Part model, mm, in its own coordinate system. A direction names the side the tool comes from. Round coordinates to 2 decimals unless told otherwise and drop trailing zeros.
```python
from build123d import *

# Parameters (mm, degrees)
F0_R     = 11.025
F1_DEPTH = 7
F2_R     = 1.5


with BuildPart() as f1:
    # F0 (on Top) → F1 (new body)
    with BuildSketch(Plane.XY):
        with BuildLine():
            Line((8.85511, 24.849853), (8.85511, 35.074853))
            Line((8.85511, 35.074853), (0, 40.187353))
            Line((0, 40.187353), (-8.85511, 35.074853))
            Line((-8.85511, 35.074853), (-8.85511, 24.849853))
            ThreePointArc((-8.85511, 24.849853), (-12.204102, 7.046041), (-25.948159, -4.756177))
            Line((-25.948159, -4.756177), (-34.803269, -9.868677))
            Line((-34.803269, -9.868677), (-34.803269, -20.093677))
            Line((-34.803269, -20.093677), (-25.948159, -25.206177))
            Line((-25.948159, -25.206177), (-17.093049, -20.093677))
            ThreePointArc((-17.093049, -20.093677), (0, -14.092083), (17.093049, -20.093677))
            Line((17.093049, -20.093677), (25.948159, -25.206177))
            Line((25.948159, -25.206177), (34.803269, -20.093677))
            Line((34.803269, -20.093677), (34.803269, -9.868677))
            Line((34.803269, -9.868677), (25.948159, -4.756177))
            ThreePointArc((25.948159, -4.756177), (12.204102, 7.046041), (8.85511, 24.849853))
        make_face()
        Polygon((-32.205193, -11.368677), (-25.948159, -7.756177), (-19.691126, -11.368677), (-19.691126, -18.593677), (-25.948159, -22.206177), (-32.205193, -18.593677), align=None, mode=Mode.SUBTRACT)
        Polygon((25.948159, -22.206177), (19.691126, -18.593677), (19.691126, -11.368677), (25.948159, -7.756177), (32.205193, -11.368677), (32.205193, -18.593677), align=None, mode=Mode.SUBTRACT)
        Circle(F0_R, mode=Mode.SUBTRACT)
        Polygon((0, 37.187353), (6.257034, 33.574853), (6.257034, 26.349853), (0, 22.737353), (-6.257034, 26.349853), (-6.257034, 33.574853), align=None, mode=Mode.SUBTRACT)
    extrude(amount=F1_DEPTH)

    # F2
    f2_edges = [f1.edges().sort_by_distance(p)[0] for p in [
        (0, -14.092083, 7),
        (-21.520604, -22.649927, 7),
        (-30.375714, -22.649927, 7),
        (-34.803269, -14.981177, 7),
        (-30.375714, -7.312427, 7),
        (-12.204102, 7.046041, 7),
        (21.520604, -22.649927, 7),
        (30.375714, -22.649927, 7),
        (34.803269, -14.981177, 7),
        (30.375714, -7.312427, 7),
        (12.204102, 7.046041, 7),
        (8.85511, 29.962353, 7),
        (4.427555, 37.631103, 7),
        (-4.427555, 37.631103, 7),
        (-8.85511, 29.962353, 7),
        (0, -14.092083, 0),
        (-21.520604, -22.649927, 0),
        (-30.375714, -22.649927, 0),
        (-34.803269, -14.981177, 0),
        (-30.375714, -7.312427, 0),
        (-12.204102, 7.046041, 0),
        (-8.85511, 29.962353, 0),
        (-4.427555, 37.631103, 0),
        (4.427555, 37.631103, 0),
        (8.85511, 29.962353, 0),
        (12.204102, 7.046041, 0),
        (30.375714, -7.312427, 0),
        (34.803269, -14.981177, 0),
        (30.375714, -22.649927, 0),
        (21.520604, -22.649927, 0),
    ]]
    fillet(f2_edges, radius=F2_R)


solid = f1.part
```
Q1. Cut at A-A on z = 2.5. State how many separate pieces and enclosed holes the cut face has, plus the area to 3 significant figures.
Values follow:
separate pieces: 1
enclosed holes: 4
area: 1,160 mm2
Q2. Mould opens along Y. For faces 1 (the flat face through (-21.583, -22.686, 3.472)), 2 (the flat face through (-19.691, -15, 3)), 3 (the flat face through (32.205, -15, 3)), 4 (the cylindrical face through (-4.28, 37.22, 6.55)) say: +Y half, -Y half, draft (parallel to the pull), parting line (faces both ways), or undercut.
Values follow:
face 1: -Y half
face 2: undercut
face 3: undercut
face 4: +Y half
Q3. Which spindle directions (+Z, -Z, +X, -X, +Y, -Y) get a long thin tool onto all of the face, cutting with end or side? Do faces 5 (the flat face through (21.459, -22.614, 3.472)), 6 (the cylindrical face through (34.376, -14.91, 6.549)), 7 (the cylindrical face through (-21.67, -22.24, 6.55)), 8 (the flat face through (-3.085, 24.518, 3.451)). Say none if no direction does.
Values follow:
face 5: +Z, -Z, -Y
face 6: +Z, +X, +Y, -Y
face 7: +Z, -Y
face 8: +Z, -Z
Q4. Wall check: L1, parallel to Y at x = 0, z = 3.25 (3 decimals); L2, parallel to X at y = -14, z = 3.25; L3, parallel to X at y = -9.5, z = 2.5. Give the ranges that are in metal, low to high.
Values follow:
L1: y = -14.092 to -11.025, 11.025 to 22.737, 37.187 to 40.187
L2: x = -34.8 to -32.21, -19.69 to 19.69, 32.21 to 34.8
L3: x = -34.16 to -28.97, -22.93 to -5.59, 5.59 to 22.93, 28.97 to 34.16
Q5. Drop flat-ended pins along their axis: pin 1 (3.5 mm diameter, centred on y = 28.5, z = 5, fed in from -X); pin 2 (1 mm diameter, centred on x = 2.5, z = 1, fed in from +Y); pin 3 (4 mm diameter, centred on x = -10, z = 3, fed in from -Y); pin 4 (8 mm diameter, centred on x = 17.5, y = 2, fed in from +Z). Give the stop position or say it passes through.
Values follow:
pin 1: stops at x = -8.86
pin 2: stops at y = 38.97
pin 3: stops at y = -16.87
pin 4: stops at z = 7
